```python
from build123d import *

# Parameters (mm, degrees)
EXTRUIR_L_MINA1_DEPTH = 100
CROQUIS2_R            = 5
CORTAR_EXTRUIR1_DEPTH = 10
CROQUIS3_R            = 7.5
CORTAR_EXTRUIR2_DEPTH = 4.5


with BuildPart() as part:
    # Croquis1 → Extruir-Lámina1 (new body)
    with BuildSketch(Plane.XY):
        Polygon((0, 125), (0, 0), (-75, 0), (-75, 10), (-10, 10), (-10, 125), align=None)
    extrude(amount=EXTRUIR_L_MINA1_DEPTH)

    # Croquis2 → Cortar-Extruir1 (cut)
    with BuildSketch(Plane(origin=(0, 0, 0), x_dir=(0, 0, -1), z_dir=(1, 0, 0))):
        with Locations((-50, 107.5)):
            Circle(CROQUIS2_R)
        with Locations((-50, 47.5)):
            Circle(CROQUIS2_R)
    extrude(amount=-CORTAR_EXTRUIR1_DEPTH, mode=Mode.SUBTRACT)

    # Croquis3 → Cortar-Extruir2 (cut)
    with BuildSketch(Plane(origin=(0, 0, 0), x_dir=(0, 0, -1), z_dir=(1, 0, 0))):
        with Locations((-50, 47.5)):
            Circle(CROQUIS3_R)
    extrude(amount=-CORTAR_EXTRUIR2_DEPTH, mode=Mode.SUBTRACT)


solid = part.part
```
Input: part model. Units: mm. Frame: model coordinates. A direction names the side the tool comes from. Round coordinates to 2 decimals unless told otherwise and drop trailing zeros. Loops run counter-clockwise (first coordinate to the right, second up) from the corner with the lowest first, then second, coordinate; pieces in that order, holes last. Notation, with made-up numbers: (22, 22) - (51, 22) arc R19 ccw to (51, 45) - close; hole circle Ø7 at (-31.75, 48.25). An arc over 180 degrees is marked (long way). One line per item, written item: value. Start each with the question number.
(1) Section B-B, the plane z = 50. Return loops of the section in (x, y).
(2) Ray query, line 1 (Z direction, x = -7, y = 47); line 2 (Y direction, x = -6.5, z = 50); line 3 (Y direction, x = -25.5, z = 73.5). Return the intervals inside material, ascending. Write a range as [from, to].
(3) Section D-D, the plane z = 78.5. Return loops of the section in (x, y).
(4) Contact query for flat-ended pins moving along their axis: P1, Ø11.5, axis at y = 47.5, z = 50, coming from the +X side; P2, Ø24, axis at y = 47.5, z = 50, coming from the -X side; P3, Ø19.5, axis at x = -32.5, z = 60, coming from the +Y side. Output: stop coordinate, or through.
(5) Section C-C, the plane y = 47.5. Return loops of the section in (x, z), plus the area to 4 significant figures.
(6) Draft query along Y for faces 1 (the flat face through (-4.5, 46, 45)), 2 (the flat face through (-5, 125, 49)), 3 (the flat face through (-9.5, 48.9, 0)). Return one class per face: +Y half, -Y half, draft (parallel to the pull), parting line (faces both ways), or undercut.
(7) Section A-A, the plane y = 107.5. Return loops of the section in (x, z).
(8) Access query for faces 4 (the flat face through (-43, 10, 49)), 5 (the cylindrical face through (-7.212, 50.879, 53.685)), 6 (the cylindrical face through (-2.22, 40.18, 51.63)). Directions: +Z, -Z, +X, -X, +Y, -Y. A direction counts if a zero-diameter tool reaches every point of the face in a straight line with its end or side. Return the directions, or none.
Results below:
1. outline: (-75, 0) - (0, 0) - (0, 40) - (-4.5, 40) - (-4.5, 42.5) - (-10, 42.5) - (-10, 10) - (-75, 10) - close; (-10, 52.5) - (-4.5, 52.5) - (-4.5, 55) - (0, 55) - (0, 102.5) - (-10, 102.5) - close; (-10, 112.5) - (0, 112.5) - (0, 125) - (-10, 125) - close
2. line 1: [0, 45.03], [54.97, 100]
2. line 2: [0, 42.5], [52.5, 102.5], [112.5, 125]
2. line 3: [0, 10]
3. outline: (-75, 0) - (0, 0) - (0, 125) - (-10, 125) - (-10, 10) - (-75, 10) - close
4. P1: x = -4.5
4. P2: x = -10
4. P3: y = 10
5. outline: (-10, 0) - (0, 0) - (0, 42.5) - (-4.5, 42.5) - (-4.5, 45) - (-10, 45) - close; (-10, 55) - (-4.5, 55) - (-4.5, 57.5) - (0, 57.5) - (0, 100) - (-10, 100) - close
5. area: 877.5 mm^2
6. face 1: undercut
6. face 2: +Y half
6. face 3: draft
7. outline: (-10, 0) - (0, 0) - (0, 45) - (-10, 45) - close; (-10, 55) - (0, 55) - (0, 100) - (-10, 100) - close
8. face 4: +Z, -Z, -X, +Y
8. face 5: +X, -X
8. face 6: +X
